Verification items for the finished model (mm, model axes). A direction names the side the tool comes from. Give positions to 0.01 mm unless a question says otherwise; leave off trailing zeros. Write each loop counter-clockwise with the first axis right and the second up, starting at its lowest first coordinate (ties: lowest second). Pieces come first, ordered by that corner, then holes. Notation, with made-up numbers: (-31.5, 48) - (-17.5, 48) arc R32 ccw to (-17.5, 84) - close; hole circle Ø8 at (-38, -34.5). An arc over 180 degrees is marked (long way). Put each result on its own line as item: value.
from build123d import *

# Parameters (mm, degrees)
SKETCH1_W           = 60
SKETCH1_H           = 3
BOSS_EXTRUDE2_DEPTH = 15
SKETCH1_5_R         = 8.13
BOSS_EXTRUDE3_DEPTH = 3
FILLET1_R           = 3
FILLET2_R           = 3


with BuildPart() as part:
    # Sketch1 → Boss-Extrude2 (new body)
    with BuildSketch(Plane.XY):
        with Locations((0, 19)):
            Rectangle(SKETCH1_W, SKETCH1_H)
    extrude(amount=BOSS_EXTRUDE2_DEPTH)

    # Sketch1<5> → Boss-Extrude3 (add)
    with BuildSketch(Plane.XY):
        with BuildLine():
            Line((30, 17.5), (-30, 17.5))
            Line((-30, 17.5), (-30, -2.5))
            ThreePointArc((-30, -2.5), (-25.606601718, -13.106601718), (-15, -17.5))
            ThreePointArc((-15, -17.5), (-4.393398282, -13.106601718), (0, -2.5))
            ThreePointArc((0, -2.5), (4.39339828, -13.106601715), (14.999999993, -17.5))
            ThreePointArc((14.999999993, -17.5), (25.606601715, -13.10660172), (30, -2.5))
            Line((30, -2.5), (30, 17.5))
        make_face()
        with Locations((-15, -2.5)):
            Circle(SKETCH1_5_R, mode=Mode.SUBTRACT)
        with Locations((15, -2.5)):
            Circle(SKETCH1_5_R, mode=Mode.SUBTRACT)
    extrude(amount=BOSS_EXTRUDE3_DEPTH)

    # Fillet1
    fillet1_edges = [part.edges().sort_by_distance(p)[0] for p in [
        (0, 17.5, 3),
    ]]
    fillet(fillet1_edges, radius=FILLET1_R)

    # Fillet2
    fillet2_edges = [part.edges().sort_by_distance(p)[0] for p in [
        (0, 20.5, 0),
    ]]
    fillet(fillet2_edges, radius=FILLET2_R)


solid = part.part
Q1. Section check B-B, the plane y = -8. Record the cut outline in (x, z).
Answers follow:
outline: (-28.96, 0) - (-20.99, 0) - (-20.99, 3) - (-28.96, 3) - close; (-9.01, 0) - (-1.04, 0) - (-1.04, 3) - (-9.01, 3) - close; (1.04, 0) - (9.01, 0) - (9.01, 3) - (1.04, 3) - close; (20.99, 0) - (28.96, 0) - (28.96, 3) - (20.99, 3) - close
Q2. Scan lines: line 1 along Y through (x, z) = (-20, 12); line 2 along Z through (x, y) = (8.5, -14); line 3 along Y through (x, z) = (15, 1.15). Record each from-to range of solid material in increasing order.
Answers follow:
line 1: y = 17.5 to 20.5
line 2: z = 0 to 3
line 3: y = -17.5 to -10.63, 5.63 to 19.86
Q3. Section check A-A, the plane y = 4.5. Record the cut outline in (x, z).
Answers follow:
outline: (-30, 0) - (-19.13, 0) - (-19.13, 3) - (-30, 3) - close; (-10.87, 0) - (10.87, 0) - (10.87, 3) - (-10.87, 3) - close; (19.13, 0) - (30, 0) - (30, 3) - (19.13, 3) - close
Q4. Section check D-D, the plane y = -0.5. Record the cut outline in (x, z).
Answers follow:
outline: (-30, 0) - (-22.88, 0) - (-22.88, 3) - (-30, 3) - close; (-7.12, 0) - (7.12, 0) - (7.12, 3) - (-7.12, 3) - close; (22.88, 0) - (30, 0) - (30, 3) - (22.88, 3) - close
Q5. Set-up check for faces 4 (the face through (0, 17.5, 10)), 5 (the face through (0, 19, 15)): record each of +Z, -Z, +X, -X, +Y, -Y from which the full face is reachable in a straight line by a thin tool's end or side.
Answers follow:
face 4: +Z, +X, -X, -Y
face 5: +Z, +X, -X, +Y, -Y
Q6. Release check for a two-part mould opening along X. For faces 1 (the face through (-21.45, -7.45, 1.48)), 2 (the face through (-30, 13, 2)), 3 (the face through (0, 2, 3)) record: released by +X, released by -X, zero draft, split by the parting line, or undercut.
Answers follow:
face 1: undercut
face 2: released by -X
face 3: zero draft
Q7. Go/stop test with flat-tipped pins: pin 1 Ø7 at (x, z) = (-14.5, 10.5) entering from -Y; pin 2 Ø14.5 at (x, y) = (15, -2.5) entering from +Z; pin 3 Ø1 at (x, y) = (5, 3.5) entering from +Z. Record where each tip stops, or that it passes through.
Answers follow:
pin 1: stops at y = 17.5
pin 2: passes through
pin 3: stops at z = 3
Q8. Section check C-C, the plane x = -3. Record the cut outline in (y, z), plus the area to 3 significant figures.
Answers follow:
outline: (-11.5, 0) - (17.5, 0) arc R3 ccw to (20.5, 3) - (20.5, 15) - (17.5, 15) - (17.5, 6) arc R3 cw to (14.5, 3) - (-11.5, 3) - close
area: 132 mm2
